```python
from build123d import *

# Parameters (mm, degrees)
SKETCH1_W               = 19.05
SKETCH1_H               = 19.05
SKETCH1_W_2             = 15.875
SKETCH1_H_2             = 15.875
TUBE_DEPTH              = 539.9532
SKETCH2_R               = 2.8956
REARWALLHOLES_DEPTH     = 20.05
LPATTERN1_COUNT         = 4
LPATTERN1_PITCH         = 156.633333333
SKETCH3_R               = 2.8956
REARTOPHOLEMASTER_DEPTH = 20.05
LPATTERN2_COUNT         = 4
LPATTERN2_PITCH         = 142.24


with BuildPart() as part:
    # Sketch1 → Tube (new body)
    with BuildSketch(Plane(origin=(0, 0, 0), x_dir=(0, -1, 0), z_dir=(1, 0, 0))):
        Rectangle(SKETCH1_W, SKETCH1_H)
        Rectangle(SKETCH1_W_2, SKETCH1_H_2, mode=Mode.SUBTRACT)
    extrude(amount=TUBE_DEPTH)

    # Sketch2 → RearWallHoles (cut, through all)
    with BuildSketch(Plane.XY.offset(9.525)):
        with Locations((504.9266, 0)):
            Circle(SKETCH2_R)
    rearwallholes = extrude(amount=-REARWALLHOLES_DEPTH, mode=Mode.SUBTRACT)

    # LPattern1: RearWallHoles ×4
    with Locations(*[(-i * LPATTERN1_PITCH, 0, 0) for i in range(1, LPATTERN1_COUNT)]):
        add(rearwallholes, mode=Mode.SUBTRACT)

    # Sketch3 → RearTopHoleMaster (cut, through all)
    with BuildSketch(Plane(origin=(0, 9.525, 0), x_dir=(1, 0, 0), z_dir=(0, 1, 0))):
        with Locations((56.6166, 0)):
            Circle(SKETCH3_R)
    reartopholemaster = extrude(amount=-REARTOPHOLEMASTER_DEPTH, mode=Mode.SUBTRACT)

    # LPattern2: RearTopHoleMaster ×4
    with Locations(*[(i * LPATTERN2_PITCH, 0, 0) for i in range(1, LPATTERN2_COUNT)]):
        add(reartopholemaster, mode=Mode.SUBTRACT)


solid = part.part
```
Geometry check sheet. Reference: the model listing, model coordinates, mm. A direction names the side the tool comes from. Coordinates: 2 decimals unless noted, no trailing zeros. Order: outer loops, then holes, each group sorted by start corner. A loop starts at its lowest first (then second) coordinate and runs counter-clockwise, first axis right, second up.
Q1. Sectioned sample at A-A on x = 415.5. Record the cut outline in (y, z) (1 decimal).
Reply:
outline: (-9.5, -9.5) - (9.5, -9.5) - (9.5, 9.5) - (-9.5, 9.5) - close; hole (-7.9, -7.9) - (7.9, -7.9) - (7.9, 7.9) - (-7.9, 7.9) - close
Q2. Draft check along Y on faces 3 (the face through (266, -9.525, 0)), 4 (the face through (0, 9, 0)), 5 (the face through (266, -7.938, 0)). Enter one of: released by +Y, released by -Y, zero draft, split by the parting line, or undercut.
Reply:
face 3: released by -Y
face 4: zero draft
face 5: undercut
Q3. Thickness scan on probe 1 along X at (y, z) = (8.7, 0); probe 2 along Y at (x, z) = (192, -1.75) (1 decimal). Record the ranges inside material, lowest first.
Reply:
probe 1: x = 0 to 53.72, 59.51 to 195.96, 201.75 to 338.2, 343.99 to 480.44, 486.23 to 539.95
probe 2: y = -9.5 to -7.9, 7.9 to 9.5
Q4. Tool access check on faces 1 (the face through (539.953, 9, 0)), 2 (the face through (266, 7.938, 0)). Record the directions out of +Z, -Z, +X, -X, +Y, -Y that give a thin tool (end or side, any length) a straight path to the whole face; none if there is none.
Reply:
face 1: +Z, -Z, +X, +Y, -Y
face 2: +X, -X
Q5. Sectioned sample at B-B on y = 0. Give the number of separate pieces and of enclosed holes in the cut face, and give its area (3 significant figures).
Reply:
separate pieces: 10
enclosed holes: 0
area: 1,640 mm2
